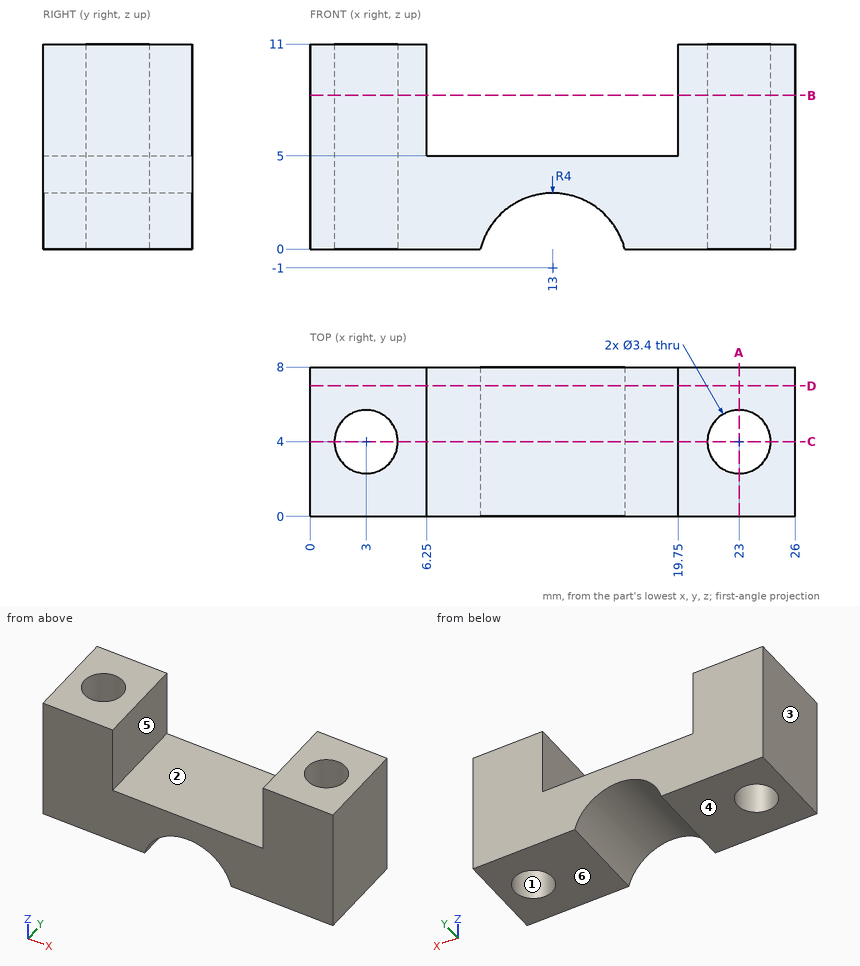
Geometry: see drawing. Coordinates: mm, zero at the bounding-box minimum. A direction names the side the tool comes from. Give positions to 0.01 mm unless a question says otherwise; leave off trailing zeros. Order: outer loops, then holes, each group sorted by start corner. A loop starts at its lowest first (then second) coordinate and runs counter-clockwise, first axis right, second up. Notation, with made-up numbers: (74, 55.25) -> (127, 55.25) arc R13 ccw to (127, 70.25) -> close; hole circle Ø5 at (50.5, -39). An arc over 180 degrees is marked (long way). Write item = value, one per line.
Q1. Cut plane B-B, the plane z = 8.25. Output: boundary loops of the cut face in (x, y).
Data:
outline = (0, 0) -> (6.25, 0) -> (6.25, 8) -> (0, 8) -> close; (19.75, 0) -> (26, 0) -> (26, 8) -> (19.75, 8) -> close; hole circle Ø3.4 at (3, 4); hole circle Ø3.4 at (23, 4)
Q2. Pin query (flat end, axial travel): pin 1 (1 mm diameter, centred on x = 18, y = 4, fed in from +Z); pin 2 (3 mm diameter, centred on x = 3, y = 4, fed in from -Z). Return the tip coordinate at first contact, or that it passes through.
Data:
pin_1 = 5
pin_2 = through
Q3. Pull-direction query (X, two-part tool) for the marked faces 1, 2, 3 and 4; classes: released by +X, released by -X, zero draft, split by the parting line, or undercut.
Data:
face_1 = undercut
face_2 = undercut
face_3 = released by -X
face_4 = zero draft
Q4. Cut plane D-D, the plane y = 7. Output: boundary loops of the cut face in (x, z), and give its area (3 significant figures).
Data:
outline = (0, 0) -> (9.13, 0) arc R4 cw to (16.87, 0) -> (26, 0) -> (26, 11) -> (19.75, 11) -> (19.75, 5) -> (6.25, 5) -> (6.25, 11) -> (0, 11) -> close
area = 188 mm^2
Q5. Set-up query: the marked faces 5 and 6. Return all of +Z, -Z, +X, -X, +Y, -Y with unobstructed straight access to the full face (end or side cutting, diameter ignored); none if empty.
Data:
face_5 = +Z, +Y, -Y
face_6 = -Z, +X, -X, +Y, -Y
Q6. Cut plane A-A, the plane x = 23. Output: boundary loops of the cut face in (y, z), and give its area (3 significant figures).
Data:
outline = (0, 0) -> (2.3, 0) -> (2.3, 11) -> (0, 11) -> close; (5.7, 0) -> (8, 0) -> (8, 11) -> (5.7, 11) -> close
area = 50.6 mm^2
Q7. Material intervals for line 1 (X direction, y = 1.5, z = 8.5); line 2 (Y direction, x = 23, z = 2.75); line 3 (X direction, y = 4.5, z = 3.5), sorted ascending. Write a range as from..to.
Data:
line_1 = 0..6.25, 19.75..26
line_2 = 0..2.3, 5.7..8
line_3 = 0..1.38, 4.62..21.38, 24.62..26
Q8. Cut plane C-C, the plane y = 4. Output: boundary loops of the cut face in (x, z), and give its area (3 significant figures).
Data:
outline = (0, 0) -> (1.3, 0) -> (1.3, 11) -> (0, 11) -> close; (4.7, 0) -> (9.13, 0) arc R4 cw to (16.87, 0) -> (21.3, 0) -> (21.3, 11) -> (19.75, 11) -> (19.75, 5) -> (6.25, 5) -> (6.25, 11) -> (4.7, 11) -> close; (24.7, 0) -> (26, 0) -> (26, 11) -> (24.7, 11) -> close
area = 113 mm^2
